from build123d import *

# Parameters (mm, degrees)
SKETCH1_R               = 1.7145
BOSS_EXTRUDE1_DEPTH     = 11.43
SKETCH2_W               = 9.906
SKETCH2_H               = 2.54
CUT_EXTRUDE1_DEPTH      = 21.259585188
CUT_EXTRUDE1_DEPTH_BACK = 21.259585188
SKETCH4_W               = 9.906
SKETCH4_H               = 20.955
SKETCH4_H_2             = 0.635
SKETCH3_R               = 1.9939
BOSS_EXTRUDE2_DEPTH     = 4.064


with BuildPart() as part:
    # Sketch1 → Boss-Extrude1 (new body)
    with BuildSketch(Plane.XY):
        with BuildLine():
            Line((-2.286, 12.234260092), (-2.286, 10.939706577))
            ThreePointArc((-2.286, 10.939706577), (-11.176, 0), (-2.286, -10.939706577))
            Line((-2.286, -10.939706577), (-2.286, -12.234260092))
            ThreePointArc((-2.286, -12.234260092), (0, -12.446), (2.286, -12.234260092))
            Line((2.286, -12.234260092), (2.286, -10.939706577))
            ThreePointArc((2.286, -10.939706577), (11.176, 0), (2.286, 10.939706577))
            Line((2.286, 10.939706577), (2.286, 12.234260092))
            ThreePointArc((2.286, 12.234260092), (0, 12.446), (-2.286, 12.234260092))
        make_face()
        Circle(SKETCH1_R, mode=Mode.SUBTRACT)
    extrude(amount=BOSS_EXTRUDE1_DEPTH)

    # Sketch2 → Cut-Revolve1 (revolve, cut)
    with BuildSketch(Plane(origin=(0, 0, 0), x_dir=(0, 0, -1), z_dir=(1, 0, 0)), mode=Mode.PRIVATE) as cut_revolve1_sk:
        with Locations((-5.715, 12.446)):
            Rectangle(SKETCH2_W, SKETCH2_H)
    revolve(cut_revolve1_sk.sketch.rotate(Axis((0, 0, 11.43), (0, 0, -1)), 348.19710831), axis=Axis((0, 0, 11.43), (0, 0, -1)), mode=Mode.SUBTRACT)

    # Sketch4 → Cut-Extrude1 (cut, two sides: drawn at the far end of the back side and taken through both)
    with BuildSketch(Plane(origin=(0, 0, 0), x_dir=(0, 0, -1), z_dir=(1, 0, 0)).offset(-CUT_EXTRUDE1_DEPTH_BACK)):
        with Locations((-5.715, 0.6985)):
            Rectangle(SKETCH4_W, SKETCH4_H)
        with Locations((-5.715, -10.8585)):
            Rectangle(SKETCH4_W, SKETCH4_H_2)
    extrude(amount=CUT_EXTRUDE1_DEPTH + CUT_EXTRUDE1_DEPTH_BACK, mode=Mode.SUBTRACT)

    # Sketch3 → Boss-Extrude2 (add)
    with BuildSketch(Plane.XY):
        with Locations((-5.477956234, 5.477956234)):
            Circle(SKETCH3_R)
    extrude(amount=BOSS_EXTRUDE2_DEPTH)


solid = part.part
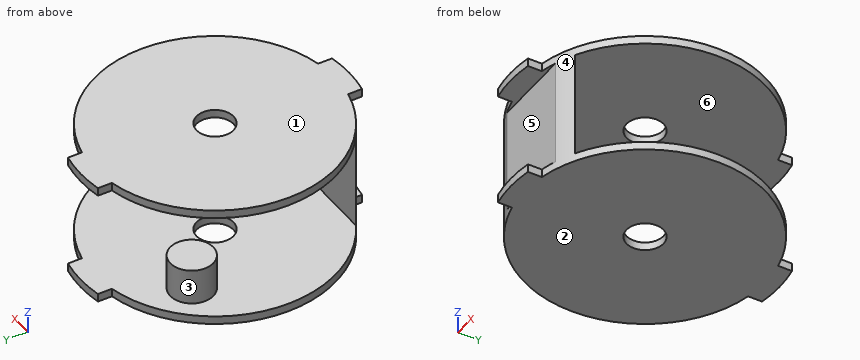
The model under review builds one solid part; all positions refer to its coordinate system, in mm. Face numbers are marked on the shaded views. A direction names the side the tool comes from. Round coordinates to 2 decimals unless told otherwise and drop trailing zeros. Write each loop counter-clockwise with the first axis right and the second up, starting at its lowest first coordinate (ties: lowest second). Pieces come first, ordered by that corner, then holes. Notation, with made-up numbers: M -38,11.5 L 1,11.5 A16 cw 1,32.5 Z; hole C -4,-0.75 d3. An arc over 180 degrees is marked long. Answer as CSV lines item,"result". Start each with the question number.
Q1. Consider section B-B, the plane y = -4.5. Give the boundary of the cut face in (x, z).
Q2. The part is to be moulded in two halves that separate along Z. For the marked faces 1, 2 and 3, say which applies: +Z half, -Z half, draft (parallel to the pull), parting line (faces both ways), or undercut.
Q3. Consider section C-C, the plane y = 0. Give the boundary of the cut face in (x, z), then the cut area to 3 significant figures.
Q4. Consider section D-D, the plane z = 6.25. Give the boundary of the cut face in (x, y), then the cut area to 3 significant figures.
Q5. Clearance check with flat-ended pins moving along their axes: P1, Ø3.5, axis at x = 1, z = 8, coming from the -Y side; P2, Ø6, axis at y = 6.5, z = 6, coming from the -X side; P3, Ø0.6, axis at x = -0.5, y = -11.5, coming from the -Z side; P4, Ø0.8, axis at y = 12, z = 0.5, coming from the +X side. State where each tip first meets the part, or that it passes through.
Q6. Wall thickness on line 1 along X through (y, z) = (0, 10.95); line 2 along Y through (x, z) = (0, 10.95); line 3 along Z through (x, y) = (-3.5, 0): over which ranges is each line inside the solid? List them lowest first.
Q7. Tool access review of the marked faces 4, 5 and 6: name each direction out of +Z, -Z, +X, -X, +Y, -Y from which nothing blocks a thin tool from reaching the whole face with its end or side.
Q8. Consider section A-A, the plane x = 0. Give the boundary of the cut face in (y, z), then the cut area to 3 significant figures.
Result set:
1,outline,"M -10.23,0 L 10.23,0 L 10.23,0.76 L -10.23,0.76 Z; M -10.23,10.67 L 10.23,10.67 L 10.23,11.43 L -10.23,11.43 Z"
2,face 1,"+Z half"
2,face 2,"-Z half"
2,face 3,"undercut"
3,outline,"M -11.18,0 L -1.71,0 L -1.71,0.76 L -11.18,0.76 Z; M -11.18,10.67 L -1.71,10.67 L -1.71,11.43 L -11.18,11.43 Z; M 1.71,0 L 11.18,0 L 11.18,0.76 L 1.71,0.76 Z; M 1.71,10.67 L 11.18,10.67 L 11.18,11.43 L 1.71,11.43 Z"
3,area,"28.8 mm²"
4,outline,"M -5.41,-9.78 A11.18 ccw -3.71,-10.54 L 3.71,-10.54 A11.18 ccw 5.41,-9.78 Z"
4,area,"7.05 mm²"
5,P1,"stops at y = -10.54"
5,P2,"stops at x = -7.47"
5,P3,"stops at z = 0"
5,P4,"stops at x = 2.29"
6,line 1,"x = -11.18 to -1.71, 1.71 to 11.18"
6,line 2,"y = -12.45 to -1.71, 1.71 to 12.45"
6,line 3,"z = 0 to 0.76, 10.67 to 11.43"
7,face 4,"+Z, -Z, +X"
7,face 5,"+X, -X, -Y"
7,face 6,"+X, -X, +Y"
8,outline,"M -12.45,0 L -1.71,0 L -1.71,0.76 L -9.78,0.76 L -9.78,10.67 L -1.71,10.67 L -1.71,11.43 L -12.45,11.43 L -12.45,10.67 L -10.54,10.67 L -10.54,0.76 L -12.45,0.76 Z; M 1.71,0 L 12.45,0 L 12.45,0.76 L 1.71,0.76 Z; M 1.71,10.67 L 12.45,10.67 L 12.45,11.43 L 1.71,11.43 Z"
8,area,"40.3 mm²"
